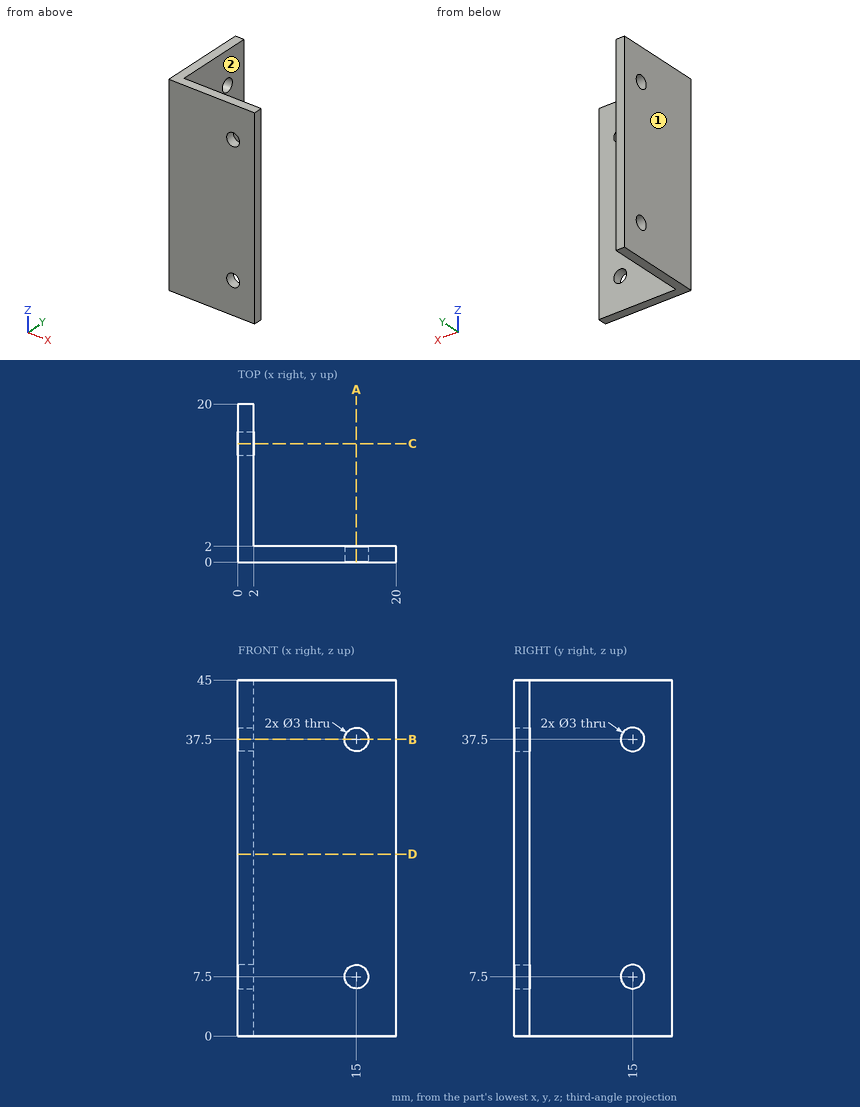
Here's the drawing with two shaded views (mm, measured from the low corner). I have some questions. A direction names the side the tool comes from. Give positions to 0.01 mm unless a question says otherwise; leave off trailing zeros. Loops run counter-clockwise (first coordinate to the right, second up) from the corner with the lowest first, then second, coordinate; pieces in that order, holes last. Notation, with made-up numbers: (9.25, 35) - (17.25, 35) arc R12 ccw to (17.25, 50) - close; hole circle Ø6 at (0.5, 7). An arc over 180 degrees is marked (long way). One line per item, written item: value.
(1) If we section it at B-B, the plane z = 37.5: List the corners of the cut face in (x, y) for me, plus the area to 3 significant figures.
Verdict:
outline: (0, 0) - (13.5, 0) - (13.5, 2) - (2, 2) - (2, 13.5) - (0, 13.5) - close; (0, 16.5) - (2, 16.5) - (2, 20) - (0, 20) - close; (16.5, 0) - (20, 0) - (20, 2) - (16.5, 2) - close
area: 64.0 mm^2
(2) If we section it at A-A, the plane x = 15: List the corners of the cut face in (y, z) for me.
Verdict:
outline: (0, 0) - (2, 0) - (2, 6) - (0, 6) - close; (0, 9) - (2, 9) - (2, 36) - (0, 36) - close; (0, 39) - (2, 39) - (2, 45) - (0, 45) - close
(3) On a 3-axis mill with a long thin cutter (end or side, diameter ignored), from which of +Z, -Z, +X, -X, +Y, -Y can I reach the whole of each face in a straight line? I mean the marked faces 1 and 2. Say none if no direction works.
Verdict:
face 1: +Z, -Z, -X, +Y, -Y
face 2: +Z, -Z, +X, +Y
(4) If we section it at D-D, the plane z = 23: List the corners of the cut face in (x, y) for me.
Verdict:
outline: (0, 0) - (20, 0) - (20, 2) - (2, 2) - (2, 20) - (0, 20) - close
(5) I'm going to push flat-ended pins straight in: pin 1 (5.5 mm diameter, centred on y = 9, z = 12.5, fed in from +X); pin 2 (4 mm diameter, centred on x = 15, z = 37.5, fed in from +Y). Where does each tip first touch, or does it pass through?
Verdict:
pin 1: x = 2
pin 2: y = 2
(6) I need wall thicknesses on line 1 along Z through (x, y) = (15, 1.45); line 2 along Y through (x, z) = (0.95, 7.5). Which ranges of each line are inside material? Lowest first, please.
Verdict:
line 1: 0 to 6, 9 to 36, 39 to 45
line 2: 0 to 13.5, 16.5 to 20
